The listing builds one solid part. Answer for the finished solid, in the listing's coordinates (mm). Face numbers are marked on the shaded views. A direction names the side the tool comes from. Give positions to 0.01 mm unless a question says otherwise; leave off trailing zeros. Order: outer loops, then holes, each group sorted by start corner. A loop starts at its lowest first (then second) coordinate and runs counter-clockwise, first axis right, second up. Notation, with made-up numbers: M 39.5,-37.5 L 98.5,-37.5 A11 cw 98.5,-27.5 Z; hole C -34,-11 d8. An arc over 180 degrees is marked long. Answer as a JSON object with one key per item and string values. Group by question number.
```python
from build123d import *

# Parameters (mm, degrees)
F0_R     = 31.75
F1_DEPTH = 53.1622
F5_D     = 9.525


with BuildPart() as f1:
    # F0 (on Front) → F1 (new body, symmetric)
    with BuildSketch(Plane.XZ):
        Circle(F0_R)
    extrude(amount=F1_DEPTH, both=True)

    # F2 (on Right) → F3 (revolve, cut)
    with BuildSketch(Plane.YZ):
        Polygon((34.925, 31.75), (0, 31.75), (0, 12.7), align=None)
        Polygon((0, 12.7), (0, 31.75), (-34.925, 31.75), align=None)
    revolve(axis=Axis((0, 0, 0), (0, 1, 0)), mode=Mode.SUBTRACT)

    # F5 (through all)
    with Locations(Plane.XZ.offset(53.1622)):
        with Locations((0, 0)):
            Hole(F5_D / 2)


solid = f1.part
```
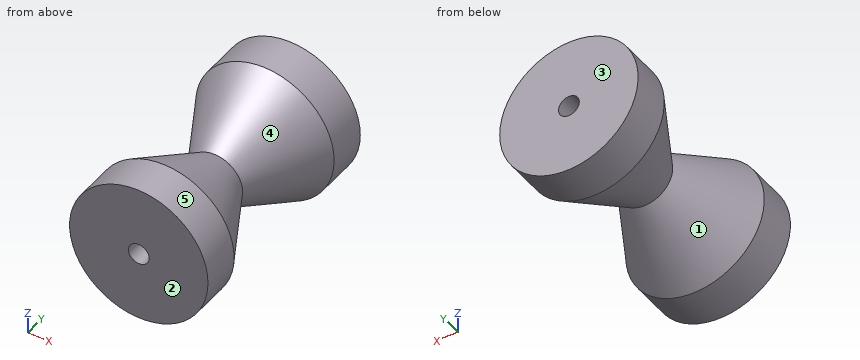
Item 1: Determine the mould class of the marked faces 1, 2 and 3 for opening direction Y: released by +Y, released by -Y, zero draft, split by the parting line, or undercut.
Item 2: Flat-ended cylindrical pins translate along their axes: P1, Ø3, axis at y = 39, z = -21, coming from the -X side; P2, Ø12, axis at y = -10.5, z = 17.5, coming from the -X side; P3, Ø12, axis at y = 36, z = 14, coming from the +X side. Find the tip coordinate at first contact, or state that the pin passes through.
Item 3: A tool of negligible diameter and unlimited length cuts with its end or side. For the marked faces 4 and 5, from which of +Z, -Z, +X, -X, +Y, -Y can it reach the whole face along a straight path? Write none if from no direction.
Item 4: Consider probe 1 along X at (y, z) = (-42, 0.5); probe 2 along Z at (x, y) = (-2.5, -18.5); probe 3 along X at (y, z) = (0, 3). Determine where each line is inside the solid, lowest interval first. Write a range as from..to.
Item 5: Section C-C (y = -27.5) is taken. Determine the outline of the cut face in (x, z) (1 decimal), and give its area (3 significant figures).
Values found:
{
 "1": {"face 1": "undercut", "face 2": "released by -Y", "face 3": "released by +Y"},
 "2": {"P1": "stops at x = -25.06", "P2": "stops at x = -15.97", "P3": "stops at x = 30.73"},
 "3": {"face 4": "none", "face 5": "+Y, -Y"},
 "4": {"probe 1": "x = -31.75..-4.74, 4.74..31.75", "probe 2": "z = -22.65..-4.05, 4.05..22.65", "probe 3": "x = -12.34..-3.7, 3.7..12.34"},
 "5": {"outline": "C 0,0 d55.4; hole C 0,0 d9.5", "area": "2,340 mm^2"}
}
